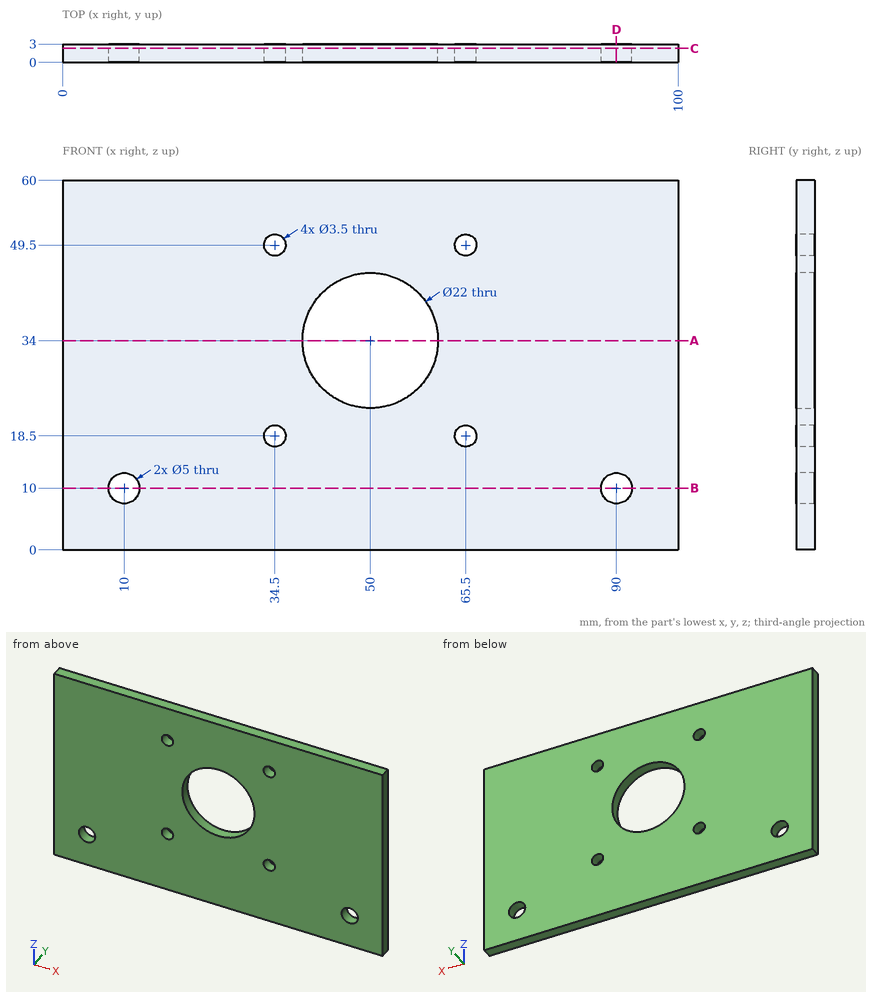
Check sheet for the drawn part. Datum: minimum x, y, z corner. Units: mm. Coordinates: 2 decimals unless noted, no trailing zeros. Order: outer loops, then holes, each group sorted by start corner. A loop starts at its lowest first (then second) coordinate and runs counter-clockwise, first axis right, second up. Notation, with made-up numbers: (89.25, 4.5) - (134.25, 4.5) arc R24 cw to (134.25, 33.5) - close; hole circle Ø11 at (48.5, -10.75). An arc over 180 degrees is marked (long way). Return JSON: item names as keys, results as strings.
(1) Section check A-A, the plane z = 34. Record the cut outline in (x, y), and give its area (3 significant figures).
Filled sheet:
{"outline": "(0, 0) - (39, 0) - (39, 3) - (0, 3) - close; (61, 0) - (100, 0) - (100, 3) - (61, 3) - close", "area": "234 mm^2"}
(2) Section check B-B, the plane z = 10. Record the cut outline in (x, y), and give its area (3 significant figures).
Filled sheet:
{"outline": "(0, 0) - (7.5, 0) - (7.5, 3) - (0, 3) - close; (12.5, 0) - (87.5, 0) - (87.5, 3) - (12.5, 3) - close; (92.5, 0) - (100, 0) - (100, 3) - (92.5, 3) - close", "area": "270 mm^2"}
(3) Section check C-C, the plane y = 2.3. Record the cut outline in (x, z).
Filled sheet:
{"outline": "(0, 0) - (100, 0) - (100, 60) - (0, 60) - close; hole circle Ø5 at (10, 10); hole circle Ø3.5 at (34.5, 18.5); hole circle Ø3.5 at (34.5, 49.5); hole circle Ø22 at (50, 34); hole circle Ø3.5 at (65.5, 18.5); hole circle Ø3.5 at (65.5, 49.5); hole circle Ø5 at (90, 10)"}
(4) Section check D-D, the plane x = 90. Record the cut outline in (y, z).
Filled sheet:
{"outline": "(0, 0) - (3, 0) - (3, 7.5) - (0, 7.5) - close; (0, 12.5) - (3, 12.5) - (3, 60) - (0, 60) - close"}
(5) Thickness scan on line 1 along Z through (x, y) = (65.5, 1.15); line 2 along X through (y, z) = (1.6, 10); line 3 along X through (y, z) = (1.3, 18.5). Record the ranges inside material, lowest first.
Filled sheet:
{"line 1": "z = 0 to 16.75, 20.25 to 47.75, 51.25 to 60", "line 2": "x = 0 to 7.5, 12.5 to 87.5, 92.5 to 100", "line 3": "x = 0 to 32.75, 36.25 to 63.75, 67.25 to 100"}
